Autodesk Inventor part; units mm, degrees
ref_plane "Work Plane1" through (150, 200.01, 1300) normal (0, 0, -1) x (-1, 0, 0)
ref_plane "Work Plane2" through (150, 200.01, 650) normal (0, 0, 1) x (1, 0, 0)
ref_plane "Work Plane3" through (0, 0, -10) normal (-1, 0, 0) x (0, 0, 1)
sketch "Sketch1" plane through (0, 0, 0) normal (0, 0, 1) x (1, 0, 0)
  circle A0 centre (0, 0) radius 15
  circle A1 centre (150, 0) radius 15
  line L0 (0, 0) -> (150, 0)
  dimension "d0" = 30
  dimension "d3" = 30
  dimension "d4" = 150
extrude "Extrusion1" add sketch "Sketch1" along normal blind 1300
sketch "Sketch2" plane through (0, 0, 0) normal (0, 1, 0) x (-1, 0, 0)
  line L0 (15, 1300) -> (-15, 1300)
  line L1 (-15, 0) -> (15, 0)
  line L2 (-135, 1300) -> (-165, 1300)
  line L3 (-165, 0) -> (-135, 0)
  circle A0 centre (0, 0) radius 15
  line L4 (-165, 0) -> (-135, 0)
  circle A1 centre (-150, 0) radius 15
  line L5 (15, 1300) -> (-15, 1300)
  circle A2 centre (0, 1300) radius 15
  line L6 (-135, 1300) -> (-165, 1300)
  circle A3 centre (-150, 1300) radius 15
extrude "Extrusion2" add sketch "Sketch2" along normal blind 200
sketch "Sketch3" plane through (0, 0, 1300) normal (0, 0, 1) x (1, 0, 0)
  line L0 (135, 0) -> (165, 0)
  line L1 (165, 0) -> (135, 0)
  arc A0 (135, 0) -> (165, 0) centre (150, 0) ccw
  line L2 (15, 0) -> (-15, 0)
  arc A1 (-15, 0) -> (15, 0) centre (0, 0) ccw
  circle A2 centre (150, 0) radius 15
  line L3 (165, 0) -> (135, 0)
  circle A3 centre (0, 0) radius 15
  line L4 (15, 0) -> (-15, 0)
revolve "Revolution1" add sketch "Sketch3" angle 90 about axis through (135, 0, 1300) along (-1, 0, 0) contours L0 A0 | A1 L2
sketch "Sketch4" plane through (0, 0, 0) normal (0, 0, -1) x (-1, 0, 0)
  line L0 (15, 0) -> (-15, 0)
  arc A0 (-15, 0) -> (15, 0) centre (0, 0) ccw
  line L1 (-135, 0) -> (-165, 0)
  arc A1 (-165, 0) -> (-135, 0) centre (-150, 0) ccw
  circle A2 centre (0, 0) radius 15
  circle A3 centre (-150, 0) radius 15
  line L2 (-165, 0) -> (-135, 0)
  line L3 (15, 0) -> (-15, 0)
revolve "Revolution2" add sketch "Sketch4" angle 90 about axis through (-15, 0, 0) along (1, 0, 0) contours A0 L0 | A1 L1
sketch "Sketch5" plane through (150, 200, 1300) normal (0, 1, 0) x (1, 0, 0)
  circle A0 centre (0, 0) radius 15
  circle A1 centre (0, 0) radius 15
  line L0 (-15, 0) -> (0, 0)
  line L1 (0, 0) -> (0, -15)
  point P0 (-150, 1300)
  point P1 (15, 0)
extrude "Extrusion4" add sketch "Sketch5" along normal blind 0.01 contours L0 L1 A0 picked at (-1.1126, -9.8746)
ref_plane "Work Plane1" through (150, 200.01, 1300) normal (0, 0, -1) x (-1, 0, 0)
sketch "Sketch6" plane through (150, 200.01, 1300) normal (0, 0, -1) x (-1, 0, 0)
  line L0 (15, -0.01) -> (-15, -0.01)
  line L1 (165, -0.01) -> (135, -0.01)
  circle A0 centre (150, -0.01) radius 15
  circle A1 centre (0, -0.01) radius 15
  point P0 (150, -200.01)
extrude "Extrusion5" add sketch "Sketch6" along normal blind 1300
ref_plane "Work Plane2" through (150, 200.01, 650) normal (0, 0, 1) x (1, 0, 0)
sketch "Sketch7" plane through (150, 200.01, 650) normal (0, 0, 1) x (1, 0, 0)
  arc A0 (15, -0.01) -> (-15, -0.01) centre (0, -0.01) ccw
  arc A1 (-15, -0.01) -> (15, -0.01) centre (0, -0.01) ccw
  line L0 (15, -0.01) -> (-15, -0.01)
  arc A2 (15, -200.01) -> (-15, -200.01) centre (0, -200.01) ccw
  line L1 (-15, -200.01) -> (15, -200.01)
  circle A3 centre (0, -0.01) radius 15
  line L2 (-165, -0.01) -> (-135, -0.01)
  arc A4 (-135, -0.01) -> (-165, -0.01) centre (-150, -0.01) ccw
  arc A5 (-165, -0.01) -> (-135, -0.01) centre (-150, -0.01) ccw
  line L3 (-135, -0.01) -> (-165, -0.01)
  arc A6 (-135, -200.01) -> (-165, -200.01) centre (-150, -200.01) ccw
  line L4 (-165, -200.01) -> (-135, -200.01)
  circle A7 centre (-150, -0.01) radius 15
extrude "Extrusion6" cut sketch "Sketch7" along normal mid plane 1225 contours L0 A0 | A1 L0 | A4 L2 | L2 A5
ref_plane "Work Plane3" through (0, 0, -10) normal (-1, 0, 0) x (0, 0, 1)
sketch "Sketch8" plane through (0, 0, -10) normal (-1, 0, 0) x (0, 0, 1)
  line L0 (1310, 0) -> (1310, 0)
  line L1 (1310, 0) -> (1310, 0)
  line L2 (10, 0) -> (10, 0)
  line L3 (10, 0) -> (10, 0)
  line L4 (10, 200) -> (10, 200)
  line L5 (10, 200) -> (10, 200)
  line L6 (10, 0) -> (10, 0)
  line L7 (10, 0) -> (10, 0)
  line L8 (25, 15) -> (1295, 15)
  line L9 (10, -15) -> (1310, -15)
  line L10 (10, 0) -> (10, -15)
  line L11 (10, 0) -> (25, 15)
  line L12 (25, 15) -> (25, 185)
  line L13 (-5, 0) -> (-5, 200)
  line L14 (-5, 0) -> (10, 0)
  line L15 (1295, 15) -> (1310, 0)
  line L16 (1310, 0) -> (1325, 0)
  line L17 (1310, -15) -> (1310, 0)
  line L18 (1325, 0) -> (1325, 200)
  line L19 (1295, 15) -> (1295, 185)
  arc A0 (1310, -15) -> (1325, 0) centre (1310, 0) ccw
  line L20 (10, 0) -> (10, 0)
  line L21 (10, 0) -> (10, 0)
  arc A1 (-5, 0) -> (10, -15) centre (10, 0) ccw
  circle A2 centre (10, 0) radius 15
  circle A3 centre (1310, 0) radius 15
extrude "Extrusion7" add sketch "Sketch8" against normal blind 150 contours A2 L10 L11 | L11 L14 A2 | A3 L16 L15 | L15 L17 A3 | L10 A1 L14 | L16 A0 L17
properties part number "Y_Rail_Bridge-Rod-Rev1"
Part model, mm, in its own coordinate system. A direction names the side the tool comes from. Coordinates: 2 decimals unless noted, no trailing zeros. Loops run counter-clockwise (first coordinate to the right, second up) from the corner with the lowest first, then second, coordinate; pieces in that order, holes last. Notation, with made-up numbers: M 5.25,37.25 L 9.25,37.25 A9 cw 9.25,44.25 Z; hole C 69,8.5 d2. An arc over 180 degrees is marked long. Use a Markdown table: item, result. Add a question column.
Q1. Probe L1, parallel to Z at x = 14.5, y = -2; L2, parallel to X at y = 12.5, z = 636; L3, parallel to Z at x = 64, y = -4. List the from-to ranges inside material, lowest first.
Q2. Which spindle directions (+Z, -Z, +X, -X, +Y, -Y) get a long thin tool onto all of the face, cutting with end or side? Do faces 3 (the cylindrical face through (-6.92, 98.6, 1313.31)), 4 (the flat face through (150, 200, 37.5)). Say none if no direction does.
Q3. Mould opens along Y. For faces 1 (the cylindrical face through (-8.06, 98.6, -12.65)), 2 (the flat face through (150, 200, 1262.5)) say: +Y half, -Y half, draft (parallel to the pull), parting line (faces both ways), or undercut.
Q4. Cut at B-B (z = 1215). Write the cut outline in (x, y).
Q5. Cut at A-A (y = 75). Write the cut outline in (x, z), and give its area (3 significant figures).
Q6. Pin check, flat tips, straight feed: P1, Ø9, axis at x = 157.5, y = 193.5, coming from the -Z side; P2, Ø16.5, axis at x = 139, z = 1305, coming from the +Y side; P3, Ø4.5, axis at x = 152, y = 211, coming from the -Z side. Stop position of each tip, or through.
Q7. Cut at C-C (x = 50.5). Write the cut outline in (y, z), and give its area (3 significant figures).
Worked out:
| question | item | result |
|---|---|---|
| 1 | L1 | z = -14.87 to 1314.87 |
| 1 | L2 | x = -8.29 to 8.29, 141.71 to 158.29 |
| 1 | L3 | z = -14.46 to 14.46, 1285.54 to 1314.46 |
| 2 | face 3 | none |
| 2 | face 4 | +X, -X, +Y |
| 3 | face 1 | undercut |
| 3 | face 2 | draft |
| 4 | outline | C 0,0 d30; C 150,0 d30 |
| 5 | outline | C 0,0 d30; C 0,1300 d30; C 150,0 d30; C 150,1300 d30 |
| 5 | area | 2,830 mm2 |
| 6 | P1 | stops at z = -14.7 |
| 6 | P2 | stops at y = 214.33 |
| 6 | P3 | stops at z = 0 |
| 7 | outline | C 0,0 d30; C 0,1300 d30 |
| 7 | area | 1,410 mm2 |
